Could you check a few things on this model? Use its own coordinates, in mm. Round coordinates to 2 decimals unless told otherwise and drop trailing zeros. Loops run counter-clockwise (first coordinate to the right, second up) from the corner with the lowest first, then second, coordinate; pieces in that order, holes last. Notation, with made-up numbers: (-24.5, 47.25) -> (-15.5, 47.25) arc R11 ccw to (-15.5, 57.25) -> close; hole circle Ø6 at (88, 80.25). An arc over 180 degrees is marked (long way). Use CSV: the item, a comma, the result in double quotes. Start each with the question number.
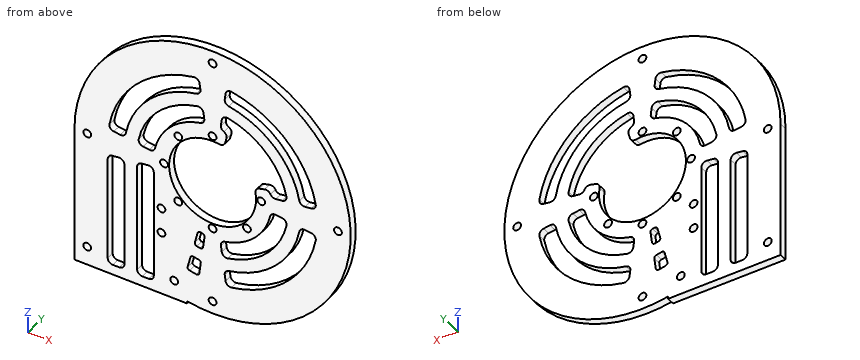
```python
from build123d import *

# Parameters (mm, degrees)
SKETCH_1_R          = 1.525
SKETCH_1_R_2        = 17
EXTRUDE_1_DEPTH     = 3
CUT_EXTRUDE_2_DEPTH = 77.426435217
CUT_EXTRUDE_3_DEPTH = 77.426435217
FILLET_1_R          = 2


with BuildPart() as part:
    # 草图1 → 凸台-拉伸1 (new body)
    with BuildSketch(Plane(origin=(0, 0, 0), x_dir=(1, 0, 0), z_dir=(0, 1, 0))):
        with BuildLine():
            Line((-54, 0), (-54, 54))
            Line((-54, 54), (-10, 54))
            Line((-10, 54), (-10, 53.065996646))
            ThreePointArc((-10, 53.065996646), (41.569219382, -34.467375879), (-54, 0))
        make_face()
        with Locations(Location((-15, 46.647615159, 0), (0, 0, 270))):
            Circle(SKETCH_1_R, mode=Mode.SUBTRACT)
        with Locations(Location((0, 49, 0), (0, 0, 270))):
            Circle(SKETCH_1_R, mode=Mode.SUBTRACT)
        with Locations(Location((49, 0, 0), (0, 0, 270))):
            Circle(SKETCH_1_R, mode=Mode.SUBTRACT)
        with Locations(Location((0, -49, 0), (0, 0, 270))):
            Circle(SKETCH_1_R, mode=Mode.SUBTRACT)
        with Locations(Location((-49, 0, 0), (0, 0, 270))):
            Circle(SKETCH_1_R, mode=Mode.SUBTRACT)
        with Locations(Location((0, 0, 0), (0, 0, 270))):
            Circle(SKETCH_1_R_2, mode=Mode.SUBTRACT)
        with Locations(Location((0, 19, 0), (0, 0, 270))):
            Circle(SKETCH_1_R, mode=Mode.SUBTRACT)
        with Locations(Location((13.435028843, 13.435028843, 0), (0, 0, 270))):
            Circle(SKETCH_1_R, mode=Mode.SUBTRACT)
        with Locations(Location((19, 0, 0), (0, 0, 270))):
            Circle(SKETCH_1_R, mode=Mode.SUBTRACT)
        with Locations(Location((13.435028843, -13.435028843, 0), (0, 0, 270))):
            Circle(SKETCH_1_R, mode=Mode.SUBTRACT)
        with Locations(Location((0, -19, 0), (0, 0, 270))):
            Circle(SKETCH_1_R, mode=Mode.SUBTRACT)
        with Locations(Location((-13.435028843, -13.435028843, 0), (0, 0, 270))):
            Circle(SKETCH_1_R, mode=Mode.SUBTRACT)
        with Locations(Location((-19, 0, 0), (0, 0, 270))):
            Circle(SKETCH_1_R, mode=Mode.SUBTRACT)
        with Locations(Location((-13.435028843, 13.435028843, 0), (0, 0, 270))):
            Circle(SKETCH_1_R, mode=Mode.SUBTRACT)
        with Locations(Location((-49, 46.647615159, 0), (0, 0, 270))):
            Circle(SKETCH_1_R, mode=Mode.SUBTRACT)
        with Locations(Location((-20, 28.979991994, 0), (0, 0, 270))):
            Circle(SKETCH_1_R, mode=Mode.SUBTRACT)
        with Locations(Location((-20, 18.979991994, 0), (0, 0, 270))):
            Circle(SKETCH_1_R, mode=Mode.SUBTRACT)
    extrude(amount=EXTRUDE_1_DEPTH)

    # 草图2 → 切除-拉伸2 (cut, through all)
    with BuildSketch(Plane(origin=(0, 0, 0), x_dir=(1, 0, 0), z_dir=(0, 1, 0))):
        with BuildLine():
            Line((-41, 7.151705327), (-41, 48))
            ThreePointArc((-41, 48), (-40.414213562, 49.414213562), (-39, 50))
            Line((-39, 50), (-36.5, 50))
            ThreePointArc((-36.5, 50), (-35.085786438, 49.414213562), (-34.5, 48))
            Line((-34.5, 48), (-34.5, 6.822574083))
            ThreePointArc((-34.5, 6.822574083), (-35.18130837, 5.318894468), (-36.761052384, 4.83968436))
            Line((-36.761052384, 4.83968436), (-39.261052384, 5.168815604))
            ThreePointArc((-39.261052384, 5.168815604), (-40.503679615, 5.833013697), (-41, 7.151705327))
        make_face()
        with BuildLine():
            Line((-23, 48), (-23, 5.308570361))
            ThreePointArc((-23, 5.308570361), (-23.68130837, 3.804890746), (-25.261052384, 3.325680638))
            Line((-25.261052384, 3.325680638), (-27.761052384, 3.654811882))
            ThreePointArc((-27.761052384, 3.654811882), (-29.003679615, 4.319009975), (-29.5, 5.637701605))
            Line((-29.5, 5.637701605), (-29.5, 48))
            ThreePointArc((-29.5, 48), (-28.914213562, 49.414213562), (-27.5, 50))
            Line((-27.5, 50), (-25, 50))
            ThreePointArc((-25, 50), (-23.585786438, 49.414213562), (-23, 48))
        make_face()
        with BuildLine():
            Line((-9.753048304, 38.779866539), (-8.655100658, 34.414230089))
            ThreePointArc((-8.655100658, 34.414230089), (-8.210625652, 33.807230719), (-7.468813536, 33.681847104))
            ThreePointArc((-7.468813536, 33.681847104), (-6.469677057, 33.887951823), (-5.464883503, 34.064424967))
            ThreePointArc((-5.464883503, 34.064424967), (-4.821436337, 34.45427367), (-4.631841062, 35.182325795))
            Line((-4.631841062, 35.182325795), (-5.219415856, 39.645399457))
            ThreePointArc((-5.219415856, 39.645399457), (-5.612064549, 40.315774725), (-6.366132236, 40.502745097))
            ThreePointArc((-6.366132236, 40.502745097), (-7.68860172, 40.272638399), (-9.002829744, 39.999363202))
            ThreePointArc((-9.002829744, 39.999363202), (-9.634981946, 39.547744349), (-9.753048304, 38.779866539))
        make_face()
        with BuildLine():
            Line((-3.71770584, 28.238779423), (-3.129908136, 23.774012599))
            ThreePointArc((-3.129908136, 23.774012599), (-3.315486635, 23.051388943), (-3.949629956, 22.65834114))
            ThreePointArc((-3.949629956, 22.65834114), (-4.313118038, 22.591967882), (-4.675492953, 22.51976389))
            ThreePointArc((-4.675492953, 22.51976389), (-5.409834137, 22.65154914), (-5.848575028, 23.25498162))
            Line((-5.848575028, 23.25498162), (-6.946939204, 27.622274267))
            ThreePointArc((-6.946939204, 27.622274267), (-6.82621795, 28.39444337), (-6.186863621, 28.843937292))
            ThreePointArc((-6.186863621, 28.843937292), (-5.532042701, 28.976654458), (-4.874384059, 29.09450773))
            ThreePointArc((-4.874384059, 29.09450773), (-4.114403615, 28.912166101), (-3.71770584, 28.238779423))
        make_face()
        with BuildLine():
            Line((5.083823439, 38.615472796), (4.757048519, 36.133370856))
            ThreePointArc((4.757048519, 36.133370856), (5.120458294, 34.698740737), (6.370626558, 33.90671198))
            ThreePointArc((6.370626558, 33.90671198), (24.395183951, 24.395183951), (33.90671198, 6.370626558))
            ThreePointArc((33.90671198, 6.370626558), (34.698740737, 5.120458294), (36.133370856, 4.757048519))
            Line((36.133370856, 4.757048519), (38.615472796, 5.083823439))
            ThreePointArc((38.615472796, 5.083823439), (39.971833872, 5.890289047), (40.321313766, 7.429108709))
            ThreePointArc((40.321313766, 7.429108709), (28.991378029, 28.991378029), (7.429108709, 40.321313766))
            ThreePointArc((7.429108709, 40.321313766), (5.890289047, 39.971833872), (5.083823439, 38.615472796))
        make_face()
        with BuildLine():
            Line((3.579964886, 27.192533008), (3.252695949, 24.706678633))
            ThreePointArc((3.252695949, 24.706678633), (3.601410919, 23.292598548), (4.816738818, 22.489976148))
            ThreePointArc((4.816738818, 22.489976148), (16.263455967, 16.263455967), (22.489976148, 4.816738818))
            ThreePointArc((22.489976148, 4.816738818), (23.292598548, 3.601410919), (24.706678633, 3.252695949))
            Line((24.706678633, 3.252695949), (27.192533008, 3.579964886))
            ThreePointArc((27.192533008, 3.579964886), (28.561439402, 4.40387472), (28.89013376, 5.967425853))
            ThreePointArc((28.89013376, 5.967425853), (20.859650045, 20.859650045), (5.967425853, 28.89013376))
            ThreePointArc((5.967425853, 28.89013376), (4.40387472, 28.561439402), (3.579964886, 27.192533008))
        make_face()
        with BuildLine():
            Line((38.615472796, -5.083823439), (36.133370856, -4.757048519))
            ThreePointArc((36.133370856, -4.757048519), (34.698740737, -5.120458294), (33.90671198, -6.370626558))
            ThreePointArc((33.90671198, -6.370626558), (24.395183951, -24.395183951), (6.370626558, -33.90671198))
            ThreePointArc((6.370626558, -33.90671198), (5.120458294, -34.698740737), (4.757048519, -36.133370856))
            Line((4.757048519, -36.133370856), (5.083823439, -38.615472796))
            ThreePointArc((5.083823439, -38.615472796), (5.890289047, -39.971833872), (7.429108709, -40.321313766))
            ThreePointArc((7.429108709, -40.321313766), (28.991378029, -28.991378029), (40.321313766, -7.429108709))
            ThreePointArc((40.321313766, -7.429108709), (39.971833872, -5.890289047), (38.615472796, -5.083823439))
        make_face()
        with BuildLine():
            Line((27.192533008, -3.579964886), (24.706678633, -3.252695949))
            ThreePointArc((24.706678633, -3.252695949), (23.292598548, -3.601410919), (22.489976148, -4.816738818))
            ThreePointArc((22.489976148, -4.816738818), (16.263455967, -16.263455967), (4.816738818, -22.489976148))
            ThreePointArc((4.816738818, -22.489976148), (3.601410919, -23.292598548), (3.252695949, -24.706678633))
            Line((3.252695949, -24.706678633), (3.579964886, -27.192533008))
            ThreePointArc((3.579964886, -27.192533008), (4.40387472, -28.561439402), (5.967425853, -28.89013376))
            ThreePointArc((5.967425853, -28.89013376), (20.859650045, -20.859650045), (28.89013376, -5.967425853))
            ThreePointArc((28.89013376, -5.967425853), (28.561439402, -4.40387472), (27.192533008, -3.579964886))
        make_face()
        with BuildLine():
            Line((-5.083823439, -38.615472796), (-4.757048519, -36.133370856))
            ThreePointArc((-4.757048519, -36.133370856), (-5.120458294, -34.698740737), (-6.370626558, -33.90671198))
            ThreePointArc((-6.370626558, -33.90671198), (-24.395183951, -24.395183951), (-33.90671198, -6.370626558))
            ThreePointArc((-33.90671198, -6.370626558), (-34.698740737, -5.120458294), (-36.133370856, -4.757048519))
            Line((-36.133370856, -4.757048519), (-38.615472796, -5.083823439))
            ThreePointArc((-38.615472796, -5.083823439), (-39.971833872, -5.890289047), (-40.321313766, -7.429108709))
            ThreePointArc((-40.321313766, -7.429108709), (-28.991378029, -28.991378029), (-7.429108709, -40.321313766))
            ThreePointArc((-7.429108709, -40.321313766), (-5.890289047, -39.971833872), (-5.083823439, -38.615472796))
        make_face()
        with BuildLine():
            Line((-3.579964886, -27.192533008), (-3.252695949, -24.706678633))
            ThreePointArc((-3.252695949, -24.706678633), (-3.601410919, -23.292598548), (-4.816738818, -22.489976148))
            ThreePointArc((-4.816738818, -22.489976148), (-16.263455967, -16.263455967), (-22.489976148, -4.816738818))
            ThreePointArc((-22.489976148, -4.816738818), (-23.292598548, -3.601410919), (-24.706678633, -3.252695949))
            Line((-24.706678633, -3.252695949), (-27.192533008, -3.579964886))
            ThreePointArc((-27.192533008, -3.579964886), (-28.561439402, -4.40387472), (-28.89013376, -5.967425853))
            ThreePointArc((-28.89013376, -5.967425853), (-20.859650045, -20.859650045), (-5.967425853, -28.89013376))
            ThreePointArc((-5.967425853, -28.89013376), (-4.40387472, -28.561439402), (-3.579964886, -27.192533008))
        make_face()
    extrude(amount=CUT_EXTRUDE_2_DEPTH, mode=Mode.SUBTRACT)

    # 草图3 → 切除-拉伸3 (cut, through all)
    with BuildSketch(Plane(origin=(0, 3, 0), x_dir=(1, 0, 0), z_dir=(0, 1, 0))):
        with BuildLine():
            Line((0, 0), (5.952838037, -22.216294005))
            ThreePointArc((5.952838037, -22.216294005), (16.263455967, -16.263455967), (22.216294005, -5.952838037))
            Line((22.216294005, -5.952838037), (0, 0))
        make_face()
    extrude(amount=-CUT_EXTRUDE_3_DEPTH, mode=Mode.SUBTRACT)

    # 圆角1
    fillet_1_edges = [part.edges().sort_by_distance(p)[0] for p in [
        (5.952838037, 1.5, 22.216294005),
        (4.399923767, 1.5, 16.420739047),
        (16.420739047, 1.5, 4.399923767),
        (22.216294005, 1.5, 5.952838037),
    ]]
    fillet(fillet_1_edges, radius=FILLET_1_R)


solid = part.part
```
1. Suppose I cut it at D-D (z = 49). List the corners of the cut face in (x, y) for me (3 decimals), then the cut area to 3 significant figures.
2. Will these pins go through, and if not, where does the flat tip stop? pin 1 (4 mm diameter, centred on x = -20, z = -18.98, fed in from -Y); pin 2 (1.5 mm diameter, centred on x = 2.5, y = 2, fed in from -Z).
3. Suppose I cut it at C-C (x = 30.5). List the corners of the cut face in (y, z) for me.
4. If I drill on L1, parallel to X at y = 0.95, z = 0 (3 decimals); L2, parallel to Z at x = 35.5, y = 0.25; L3, parallel to X at y = 0.65, z = -6.5, over which ranges is the centre line in solid material (lowest first)?
5. Suppose I cut it at B-B (x = 49). List the corners of the cut face in (y, z) for me (3 decimals).
6. Suppose I cut it at A-A (z = -42). List the corners of the cut face in (x, y) for me, then the cut area to 3 significant figures.
Geometry check:
1,outline,"(-22.694, 0) -> (-1.525, 0) -> (-1.525, 3) -> (-22.694, 3) -> close; (1.525, 0) -> (22.694, 0) -> (22.694, 3) -> (1.525, 3) -> close"
1,area,"127 mm²"
2,pin 1,"stops at y = 0"
2,pin 2,"stops at z = -53.97"
3,outline,"(0, -44.56) -> (3, -44.56) -> (3, -27.4) -> (0, -27.4) -> close; (0, -16.12) -> (3, -16.12) -> (3, 16.12) -> (0, 16.12) -> close; (0, 27.4) -> (3, 27.4) -> (3, 44.56) -> (0, 44.56) -> close"
4,L1,"x = -54 to -50.525, -47.475 to -20.525, -17.475 to -17, 17 to 17.475, 20.525 to 47.475, 50.525 to 54"
4,L2,"z = -40.69 to -20.51, -4.77 to 4.77, 20.51 to 40.69"
4,L3,"x = -54 to -40.89, -34.53 to -29.5, -23 to -15.71, 15.71 to 22.06, 28.77 to 33.88, 40.27 to 53.61"
5,outline,"(0, -22.694) -> (3, -22.694) -> (3, -1.525) -> (0, -1.525) -> close; (0, 1.525) -> (3, 1.525) -> (3, 22.694) -> (0, 22.694) -> close"
6,outline,"(-54, 0) -> (-41, 0) -> (-41, 3) -> (-54, 3) -> close; (-34.5, 0) -> (-29.5, 0) -> (-29.5, 3) -> (-34.5, 3) -> close; (-23, 0) -> (33.94, 0) -> (33.94, 3) -> (-23, 3) -> close"
6,area,"225 mm²"
